from build123d import *

# Parameters (mm, degrees)
SKETCH1_R           = 1.75
BOSS_EXTRUDE1_DEPTH = 2
SCALE1_DEPTH        = 2
SCALE1_START        = -0.999997816
SCALE1_2_OUTLINE_R  = 3.5
SCALE1_2_DEPTH      = 4


# Read off the part's stored shape, not the designer's step: Scale1
with BuildPart() as part:
    # Sketch1 → Boss-Extrude1 (new body)
    with BuildSketch(Plane.XY):
        with BuildLine():
            Line((37.774530777, -2.80976251), (26.258490635, -9.838609559))
            ThreePointArc((26.258490635, -9.838609559), (23.654335286, -10.570760941), (21.04996396, -9.839378194))
            Line((21.04996396, -9.839378194), (0, 3))
            ThreePointArc((0, 3), (-2.885775614, -0.819938477), (1.577438975, -2.551800596))
            Line((1.577438975, -2.551800596), (2.923005699, -1.720015621))
            Line((2.923005699, -1.720015621), (27.42442319, -16.619165126))
            ThreePointArc((27.42442319, -16.619165126), (28.420022181, -17.142817893), (29.530314816, -17.323593546))
            Line((29.530314816, -17.323593546), (36.531170313, -17.323593546))
            ThreePointArc((36.531170313, -17.323593546), (36.747003069, -17.316932382), (36.962014284, -17.296974244))
            Line((36.962014284, -17.296974244), (42.4263802, -16.619165126))
            add(Edge.make_bspline(
                [(37.774530777, -2.80976251), (45.652503852, 1.576646515), (46.016818074, -16.230167124), (42.4263802, -16.619165126)],
                knots=[0, 0, 0, 0, 1, 1, 1, 1], degree=3))
        make_face()
        Circle(SKETCH1_R, mode=Mode.SUBTRACT)
        with Locations((40, -13.83)):
            Circle(SKETCH1_R, mode=Mode.SUBTRACT)
        with BuildLine():
            ThreePointArc((40, -7.58), (41.75, -5.83), (40, -4.08))
            ThreePointArc((40, -4.08), (33.105708883, -6.935708883), (30.25, -13.83))
            ThreePointArc((30.25, -13.83), (32, -15.58), (33.75, -13.83))
            ThreePointArc((33.75, -13.83), (35.580582618, -9.410582618), (40, -7.58))
        make_face(mode=Mode.SUBTRACT)
    extrude(amount=BOSS_EXTRUDE1_DEPTH)

    # Scale1 outline → Scale1 (cut)
    with BuildSketch(Plane.XY):
        with BuildLine():
            Line((25.309397888, -10.313026346), (25.407923969, -10.252890679))
            ThreePointArc((25.407923969, -10.252890679), (23.18128534, -10.548403138), (21.04996396, -9.839378194))
            Line((21.04996396, -9.839378194), (0, 3))
            ThreePointArc((0, 3), (-1.910769589, 2.312781783), (-2.946128732, 0.565973052))
            Line((-2.946128732, 0.565973052), (-1.741862619, -0.168566356))
            ThreePointArc((-1.741862619, -0.168566356), (0.911271712, 1.494016019), (0.647354046, -1.62586369))
            Line((0.647354046, -1.62586369), (1.869458664, -2.371283654))
            Line((1.869458664, -2.371283654), (2.923005699, -1.720015621))
            Line((2.923005699, -1.720015621), (19.42459166, -11.75452062))
            ThreePointArc((19.42459166, -11.75452062), (22.478792733, -11.490181349), (25.309397888, -10.313026346))
        make_face()
        with BuildLine():
            add(Edge.make_bspline(
                [(41.45450238, -2.430697688), (43.278912085, -3.340053045), (44.251250713, -6.082636591), (44.527913808, -8.917748085)],
                knots=[0.188633601, 0.188633601, 0.188633601, 0.188633601, 0.541520813, 0.541520813, 0.541520813, 0.541520813], degree=3))
            ThreePointArc((41.45450238, -2.430697688), (40.4125829, -3.229629308), (39.426788196, -4.096864419))
            ThreePointArc((39.426788196, -4.096864419), (39.713270083, -4.084217017), (40, -4.08))
            ThreePointArc((40, -4.08), (41.75, -5.83), (40, -7.58))
            ThreePointArc((40, -7.58), (37.394812966, -8.148846903), (35.263850756, -9.751839835))
            ThreePointArc((35.263850756, -9.751839835), (33.906901167, -13.439130778), (33.316667581, -17.323593546))
            Line((33.316667581, -17.323593546), (36.531170313, -17.323593546))
            ThreePointArc((36.531170313, -17.323593546), (36.747003069, -17.316932382), (36.962014284, -17.296974244))
            Line((36.962014284, -17.296974244), (40.373564213, -16.873799866))
            ThreePointArc((40.373564213, -16.873799866), (40.47496583, -16.16733217), (40.616522643, -15.467803355))
            ThreePointArc((40.616522643, -15.467803355), (38.347783736, -13.253214584), (41.501863894, -12.931721176))
            ThreePointArc((41.501863894, -12.931721176), (42.811031733, -10.771051035), (44.527913808, -8.917748085))
        make_face()
    extrude(amount=SCALE1_DEPTH, mode=Mode.SUBTRACT)

    # Scale1 2 outline → Scale1 2 (add)
    with BuildSketch(Plane.XY.offset(SCALE1_START)):
        with BuildLine():
            add(Edge.make_bspline(
                [(48.341478172, 3.744667751), (64.097424322, 12.517485802), (64.826052766, -23.096141476), (57.645177019, -23.874137481)],
                knots=[0, 0, 0, 0, 1, 1, 1, 1], degree=3))
            Line((48.341478172, 3.744667751), (25.309397888, -10.313026346))
            ThreePointArc((25.309397888, -10.313026346), (20.101087191, -11.77732911), (14.892344539, -10.314563616))
            Line((14.892344539, -10.314563616), (-27.207583382, 15.364192772))
            ThreePointArc((-27.207583382, 15.364192772), (-32.97913461, 7.724315817), (-24.052705432, 4.26059158))
            Line((-24.052705432, 4.26059158), (-21.361571984, 5.924161529))
            Line((-21.361571984, 5.924161529), (27.641262999, -23.874137481))
            ThreePointArc((27.641262999, -23.874137481), (29.632460981, -24.921443014), (31.85304625, -25.28299432))
            Line((31.85304625, -25.28299432), (45.854757245, -25.28299432))
            ThreePointArc((45.854757245, -25.28299432), (46.286422756, -25.269671992), (46.716445185, -25.229755716))
            Line((46.716445185, -25.229755716), (57.645177019, -23.874137481))
        make_face()
        with BuildLine():
            ThreePointArc((33.292416618, -18.295807228), (39.003834385, -4.507224995), (52.792416618, 1.204192772))
            ThreePointArc((52.792416618, 1.204192772), (56.292416618, -2.295807228), (52.792416618, -5.795807228))
            ThreePointArc((52.792416618, -5.795807228), (43.953581853, -9.456972464), (40.292416618, -18.295807228))
            ThreePointArc((40.292416618, -18.295807228), (36.792416618, -21.795807228), (33.292416618, -18.295807228))
        make_face(mode=Mode.SUBTRACT)
        with Locations((52.792416618, -18.295807228)):
            Circle(SCALE1_2_OUTLINE_R, mode=Mode.SUBTRACT)
        with Locations((-27.207583382, 9.364192772)):
            Circle(SCALE1_2_OUTLINE_R, mode=Mode.SUBTRACT)
    extrude(amount=SCALE1_2_DEPTH)


solid = part.part
Verification items for the finished model (mm, model axes). A direction names the side the tool comes from. Give positions to 0.01 mm unless a question says otherwise; leave off trailing zeros. Order: outer loops, then holes, each group sorted by start corner. A loop starts at its lowest first (then second) coordinate and runs counter-clockwise, first axis right, second up. Notation, with made-up numbers: M 46,-16.5 L 68,-16.5 A18 cw 68,16.5 Z; hole C 47,39.25 d8. An arc over 180 degrees is marked long. Answer as a JSON object with one key per item and string values. Group by question number.
1) Cross-section at C-C (y = -3.5). Give the number of separate pieces and of enclosed holes in the cut face, then the cut area to 3 significant figures.
2) Depth check by flat-ended pin: pin 1 Ø6.5 at (x, y) = (52.79, -18.3) entering from -Z; pin 2 Ø1 at (x, z) = (-12, 0) entering from -Y; pin 3 Ø1 at (y, z) = (-3, -0.5) entering from -X; pin 4 Ø1 at (y, z) = (-14, 1) entering from +X. Enter the tip coordinate at first touch or a pass-through.
3) Access from +Z, -Z, +X, -X, +Y, -Y to the whole of each face (thin tool, end or side, straight path). Record for faces 1 (the face through (-22.73, 5.08, 0.97)), 2 (the face through (56.29, -2.22, 0.97)), 3 (the face through (27, -12, 3)).
4) Mould release check, pull along Y, two halves, no side actions. Record for faces 4 (the face through (38.85, -4.66, 0.97)), 5 (the face through (-33.02, 7.87, 0.97)), 6 (the face through (27, -12, -1)): released by +Y, released by -Y, zero draft, split by the parting line, or undercut.
5) Cross-section at A-A (x = 34.5). Enter the section's corners in (y, z), then the cut area to 3 significant figures.
6) Scan lines: line 1 along X through (y, z) = (-7, 1.45); line 2 along X through (y, z) = (-10, 0.8); line 3 along Y through (x, z) = (50, 2.3). Record each from-to range of solid material in increasing order. Write a range as [from, to].
7) Cross-section at B-B (y = 8). Enter the section's corners in (x, z), then the cut area to 3 significant figures.
8) Cross-section at D-D (x = 22.5). Enter the section's corners in (y, z).
Result sheet:
{
 "1": {"separate pieces": "3", "enclosed holes": "0", "area": "72.3 mm2"},
 "2": {"pin 1": "passes through", "pin 2": "stops at y = -0.07", "pin 3": "stops at x = -7.51", "pin 4": "stops at x = 61.98"},
 "3": {"face 1": "+Z, -Z, -Y", "face 2": "+Z, -Z", "face 3": "+Z, +X, -X, +Y, -Y"},
 "4": {"face 4": "undercut", "face 5": "split by the parting line", "face 6": "zero draft"},
 "5": {"outline": "M -25.28,-1 L -20.94,-1 L -20.94,3 L -25.28,3 Z; M -11.54,-1 L -4.7,-1 L -4.7,3 L -11.54,3 Z", "area": "44.7 mm2"},
 "6": {"line 1": "x = [-0.11, 9.46], [30.74, 36.9], [47.44, 61.67]", "line 2": "x = [4.83, 14.38], [25.82, 35.15], [43.44, 61.96]", "line 3": "y = [-24.82, -20.41], [-16.19, -6.11], [1, 4.53]"},
 "7": {"outline": "M -33.05,-1 L -30.43,-1 L -30.43,3 L -33.05,3 Z; M -23.98,-1 L -15.13,-1 L -15.13,3 L -23.98,3 Z", "area": "45.9 mm2"},
 "8": {"outline": "M -20.75,-1 L -11.48,-1 L -11.48,3 L -20.75,3 Z"}
}
